from build123d import *

# Parameters (mm, degrees)
SKETCH_1_R               = 65
EXTRUDE_1_DEPTH          = 5
SKETCH_2_R               = 65
SKETCH_2_R_2             = 46.5
EXTRUDE_2_DEPTH          = 21.3
SKETCH_3_R               = 2.1
CUT_EXTRUDE_1_DEPTH      = 21.3
SKETCH_4_R               = 37.5
CUT_EXTRUDE_2_DEPTH      = 21.3
CUT_EXTRUDE_3_DEPTH      = 15
CUT_EXTRUDE_4_DEPTH      = 95.359366255
CUT_EXTRUDE_4_DEPTH_BACK = 95.359366255
SKETCH_6_R               = 2.15
CUT_EXTRUDE_START        = -1
CUT_EXTRUDE_5_DEPTH      = 1


with BuildPart() as part:
    # 草图1 → 凸台-拉伸1 (new body)
    with BuildSketch(Plane.XY):
        Circle(SKETCH_1_R)
    extrude(amount=EXTRUDE_1_DEPTH)

    # 草图2 → 凸台-拉伸2 (add)
    with BuildSketch(Plane.XY.offset(5)):
        Circle(SKETCH_2_R)
        Circle(SKETCH_2_R_2, mode=Mode.SUBTRACT)
    extrude(amount=EXTRUDE_2_DEPTH)

    # 草图3 → 切除-拉伸1 (cut)
    with BuildSketch(Plane.XY.offset(5)):
        with Locations((0, 42.5)):
            Circle(SKETCH_3_R)
        with Locations((30.0520382, 30.0520382)):
            Circle(SKETCH_3_R)
        with Locations((42.5, 0)):
            Circle(SKETCH_3_R)
        with Locations((30.0520382, -30.0520382)):
            Circle(SKETCH_3_R)
        with Locations((0, -42.5)):
            Circle(SKETCH_3_R)
        with Locations((-30.0520382, -30.0520382)):
            Circle(SKETCH_3_R)
        with Locations((-42.5, 0)):
            Circle(SKETCH_3_R)
        with Locations((-30.0520382, 30.0520382)):
            Circle(SKETCH_3_R)
    extrude(amount=-CUT_EXTRUDE_1_DEPTH, mode=Mode.SUBTRACT)

    # 草图4 → 切除-拉伸2 (cut)
    with BuildSketch(Plane(origin=(0, 0, 0), x_dir=(-1, 0, 0), z_dir=(0, 0, -1))):
        Circle(SKETCH_4_R)
    extrude(amount=-CUT_EXTRUDE_2_DEPTH, mode=Mode.SUBTRACT)

    # 草图5 → 切除-拉伸3 (cut)
    with BuildSketch(Plane(origin=(0, 0, 0), x_dir=(-1, 0, 0), z_dir=(0, 0, -1))):
        Polygon((34.449558984, 57.03733322), (19.236184468, 20.308998132), (0.758593817, 27.96266678), (15.971968334, 64.691001868), align=None)
    extrude(amount=-CUT_EXTRUDE_3_DEPTH, mode=Mode.SUBTRACT)

    # 草图6 → 切除-拉伸4 (cut, two sides: drawn at the far end of the back side and taken through both)
    with BuildSketch(Plane.XY.offset(5).offset(-CUT_EXTRUDE_4_DEPTH_BACK)):
        with Locations((0, 55)):
            Circle(SKETCH_6_R)
        with Locations((27.5, 47.631397208)):
            Circle(SKETCH_6_R)
        with Locations((47.631397208, 27.5)):
            Circle(SKETCH_6_R)
        with Locations((55, 0)):
            Circle(SKETCH_6_R)
        with Locations((47.631397208, -27.5)):
            Circle(SKETCH_6_R)
        with Locations((27.5, -47.631397208)):
            Circle(SKETCH_6_R)
        with Locations((0, -55)):
            Circle(SKETCH_6_R)
        with Locations((-27.5, -47.631397208)):
            Circle(SKETCH_6_R)
        with Locations((-47.631397208, -27.5)):
            Circle(SKETCH_6_R)
        with Locations((-55, 0)):
            Circle(SKETCH_6_R)
        with Locations((-47.631397208, 27.5)):
            Circle(SKETCH_6_R)
        with Locations(Location((-27.5, 47.631397208, 0), (0, 0, 180))):
            Circle(SKETCH_6_R)
    extrude(amount=CUT_EXTRUDE_4_DEPTH + CUT_EXTRUDE_4_DEPTH_BACK, mode=Mode.SUBTRACT)

    # 草图7 → 切除-拉伸5 (cut)
    with BuildSketch(Plane.XY.offset(5).offset(CUT_EXTRUDE_START)):
        with BuildLine():
            Line((-23.069770834, 29.564094332), (-26.617216434, 38.128385611))
            ThreePointArc((-26.617216434, 38.128385611), (17.794779605, -42.960398262), (-8.139625784, 45.782054258))
            Line((-8.139625784, 45.782054258), (-4.592180184, 37.217762979))
            ThreePointArc((-4.592180184, 37.217762979), (14.350628714, -34.645482469), (-23.069770834, 29.564094332))
        make_face()
    extrude(amount=CUT_EXTRUDE_5_DEPTH, mode=Mode.SUBTRACT)


solid = part.part
CAD build for the part. Positions are in the model's coordinates, mm. A direction names the side the tool comes from. Round coordinates to 2 decimals unless told otherwise and drop trailing zeros. Write each loop counter-clockwise with the first axis right and the second up, starting at its lowest first coordinate (ties: lowest second). Pieces come first, ordered by that corner, then holes. Notation, with made-up numbers: (20, 27.25) -> (37, 27.25) arc R31 ccw to (37, 51.25) -> close; hole circle Ø9 at (-4, 42). An arc over 180 degrees is marked (long way). Answer as a JSON object with one key per item and string values.
(1) Probe probe 1 along Y at (x, z) = (0, 2.5); probe 2 along Y at (x, z) = (0, 18.75); probe 3 along Y at (x, z) = (-27.5, 9.5). List the from-to ranges inside material, lowest first. Write a range as [from, to].
Reported:
{"probe 1": "y = [-65, -57.15], [-52.85, -44.6], [-40.4, -37.5], [37.5, 40.4], [44.6, 52.85], [57.15, 65]", "probe 2": "y = [-65, -57.15], [-52.85, -46.5], [46.5, 52.85], [57.15, 65]", "probe 3": "y = [-58.9, -49.78], [-45.48, -37.5], [37.5, 40.26]"}
(2) Band-saw the part on A-A, the plane x = 9. List the corners of the cut face in (y, z), then the cut area to 3 significant figures.
Reported:
{"outline": "(-64.37, 0) -> (-36.4, 0) -> (-36.4, 4) -> (-45.62, 4) -> (-45.62, 26.3) -> (-64.37, 26.3) -> close; (36.4, 0) -> (64.37, 0) -> (64.37, 26.3) -> (45.62, 26.3) -> (45.62, 4) -> (36.4, 4) -> close", "area": "1,060 mm^2"}
(3) Pin check, flat tips, straight feed: P1, Ø12, axis at x = -45.5, y = 45, coming from the -Z side; P2, Ø1.5, axis at x = 39.5, y = -1, coming from the +Z side; P3, Ø3, axis at x = 13, z = 11, coming from the -Y side; P4, Ø10, axis at y = 36.5, z = 15, coming from the +X side. Stop position of each tip, or through.
Reported:
{"P1": "stops at z = 0", "P2": "stops at z = 4", "P3": "stops at y = -63.97", "P4": "stops at x = 56.86"}
(4) Band-saw the part on B-B, the plane y = -34. List the corners of the cut face in (x, z).
Reported:
{"outline": "(-55.4, 0) -> (-15.82, 0) -> (-15.82, 4) -> (-31.72, 4) -> (-31.72, 26.3) -> (-55.4, 26.3) -> close; (15.82, 0) -> (55.4, 0) -> (55.4, 26.3) -> (31.72, 26.3) -> (31.72, 4) -> (15.82, 4) -> close"}
(5) Two-plate mould, pull along Y, no slides. Class faces 4 (the face through (28, -28, 0)), 5 (the face through (-29.71, 45.6, 7.4)), 6 (the face through (49.62, -28.32, 12.97)): +Y half, -Y half, draft (parallel to the pull), parting line (faces both ways), or undercut.
Reported:
{"face 4": "draft", "face 5": "+Y half", "face 6": "undercut"}
(6) Band-saw the part on C-C, the plane z = 24.5. Count the separate pieces of the cut face and the enclosed holes in it, then the cut area to 3 significant figures.
Reported:
{"separate pieces": "1", "enclosed holes": "13", "area": "6,310 mm^2"}
(7) Which spindle directions (+Z, -Z, +X, -X, +Y, -Y) get a long thin tool onto all of the face, cutting with end or side? Do faces 1 (the face through (-11.085, 52.892, 7.395)), 2 (the face through (0, -38, 4)), 3 (the face through (-28.66, 45.82, 20.57)). Say none if no direction does.
Reported:
{"face 1": "-Z", "face 2": "+Z", "face 3": "+Z, -Z"}
